The model under review builds one solid part; all positions refer to its coordinate system, in mm. Face numbers are marked on the shaded views. Coordinates: 2 decimals unless noted, no trailing zeros. Write each loop counter-clockwise with the first axis right and the second up, starting at its lowest first coordinate (ties: lowest second). Pieces come first, ordered by that corner, then holes. Notation, with made-up numbers: M 61.25,-12 L 85.25,-12 A33 cw 85.25,18 Z; hole C 82,20.5 d11. An arc over 180 degrees is marked long. Answer as a JSON object with one key per item and string values.
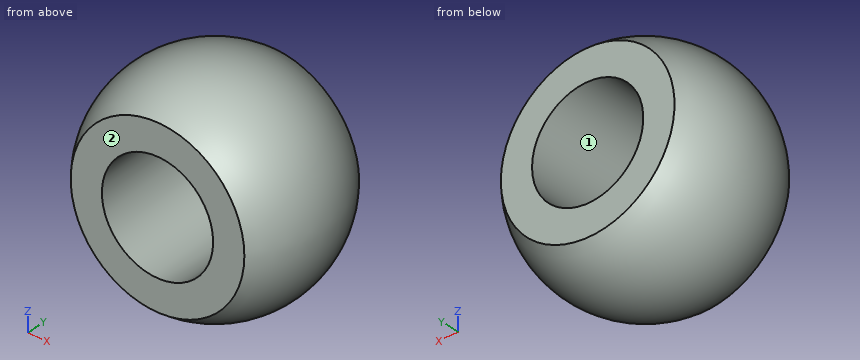
Autodesk Inventor part; units mm, degrees
ref_plane "YZ Plane" through (0, 0, 0) normal (1, 0, 0) x (0, 1, 0)
ref_plane "XZ Plane" through (0, 0, 0) normal (0, 1, 0) x (-1, 0, 0)
ref_plane "XY Plane" through (0, 0, 0) normal (0, 0, 1) x (1, 0, 0)
sketch "Sketch1" plane through (0, 0, 0) normal (0, 0, 1) x (1, 0, 0)
  arc A0 (0, -3.2) -> (0, 3.2) centre (0, 0) ccw
  line L0 (0, 3.2) -> (0, -3.2)
  dimension "d0" = 6.4
revolve "Revolution1" add sketch "Sketch1" angle 360 about axis through (0, 3.2, 0) along (0, -1, 0)
sketch "Sketch2" plane through (0, 0, 0) normal (1, 0, 0) x (0, 1, 0)
  line L0 (2, 8.8306) -> (-2, 8.8306)
  line L1 (-2, 8.8306) -> (-2, -8.8306)
  line L2 (-2, -8.8306) -> (2, -8.8306)
  line L3 (2, -8.8306) -> (2, 8.8306)
  line L4 (2, 8.8306) -> (-2, -8.8306) construction
  line L5 (-2, 8.8306) -> (2, -8.8306) construction
  line L6 (6.1175, 19.2226) -> (-9.7521, 19.2226)
  line L7 (-9.7521, 19.2226) -> (-9.7521, -16.6118)
  line L8 (-9.7521, -16.6118) -> (6.1175, -16.6118)
  line L9 (6.1175, -16.6118) -> (6.1175, 19.2226)
  point P0 (0, 0)
  dimension "d2" = 4
extrude "Extrusion1" cut sketch "Sketch2" along normal through all both and the other way through all
sketch "Sketch3" plane through (0, -2, 0) normal (0, -1, 0) x (1, 0, 0)
  circle A0 centre (0, 0) radius 2.498
  circle A1 centre (0, 0) radius 1.6
  dimension "d5" = 3.2
extrude "Extrusion2" cut sketch "Sketch3" against normal through all contours A1
properties part number "500-109" material "Aluminum 6061"
(1) Wall thickness on line 1 along Z through (x, y) = (0, 0.8); line 2 along Z through (x, y) = (-0.5, -1.7); line 3 along X through (y, z) = (0.2, 0.5): over which ranges is each line inside the solid? List them lowest first. Write a range as from..to.
Results list:
{"line 1": "-3.1..-1.6, 1.6..3.1", "line 2": "-2.66..-1.52, 1.52..2.66", "line 3": "-3.15..-1.52, 1.52..3.15"}
(2) For pin 1 Ø1.5 at (y, z) = (-1, 0) entering from +X; pin 2 Ø1 at (y, z) = (-1, -1.5) entering from -X; pin 3 Ø2 at (y, z) = (1.5, -1.5) entering from +X, all flat-tipped, find the tip position at first contact; note any pin that passes through.
Results list:
{"pin 1": "x = 3.19", "pin 2": "x = -2.92", "pin 3": "x = 3"}
(3) Add section B-B on z = 0. Give the boundary of the cut face in (x, y), and give its area (3 significant figures).
Results list:
{"outline": "M -2.5,-2 L -1.6,-2 L -1.6,2 L -2.5,2 A3.2 ccw Z; M 1.6,-2 L 2.5,-2 A3.2 ccw 2.5,2 L 1.6,2 Z", "area": "11.0 mm²"}
(4) Add section D-D on z = 2. Give the boundary of the cut face in (x, y), and give its area (3 significant figures).
Results list:
{"outline": "M -1.5,-2 L 1.5,-2 A2.5 ccw 1.5,2 L -1.5,2 A2.5 ccw Z", "area": "17.6 mm²"}
(5) Add section A-A on x = 0. Give the boundary of the cut face in (y, z).
Results list:
{"outline": "M -2,-2.5 A3.2 ccw 2,-2.5 L 2,-1.6 L -2,-1.6 Z; M -2,1.6 L 2,1.6 L 2,2.5 A3.2 ccw -2,2.5 Z"}
(6) Add section C-C on y = -0.6. Give the boundary of the cut face in (x, z).
Results list:
{"outline": "C 0,0 d6.29; hole C 0,0 d3.2"}
(7) Draft analysis for pull direction Z (two halves, no side actions). For the marked faces 1 and 2, state which applies: released by +Z, released by -Z, zero draft, split by the parting line, or undercut.
Results list:
{"face 1": "undercut", "face 2": "zero draft"}
